from build123d import *

# Parameters (mm, degrees)
SKETCH_W        = 55
SKETCH_H        = 20
PAD_DEPTH       = 10
SKETCH001_W     = 50.5
SKETCH001_H     = 4.5
POCKET_DEPTH    = 18
SKETCH002_R     = 2.5
POCKET001_DEPTH = 5
SKETCH003_W     = 10
SKETCH003_H     = 10
PAD001_DEPTH    = 80
SKETCH004_W     = 10
SKETCH004_H     = 5
PAD002_DEPTH    = 13
SKETCH005_W     = 10
SKETCH005_H     = 5
PAD003_DEPTH    = 13
SKETCH006_W     = 5
SKETCH006_H     = 5
PAD004_DEPTH    = 23
SKETCH007_W     = 5
SKETCH007_H     = 5
PAD005_DEPTH    = 23
SKETCH008_W     = 5
SKETCH008_H     = 5
PAD006_DEPTH    = 15
SKETCH009_W     = 5
SKETCH009_H     = 5
PAD007_DEPTH    = 15


with BuildPart() as part:
    # Sketch → Pad (new body)
    with BuildSketch(Plane.XY):
        Rectangle(SKETCH_W, SKETCH_H)
    extrude(amount=PAD_DEPTH)

    # Sketch001 (on Face3 of Pad) → Pocket (cut)
    with BuildSketch(Plane.XZ.offset(10)):
        with Locations((0, 5.069511)):
            Rectangle(SKETCH001_W, SKETCH001_H)
    extrude(amount=-POCKET_DEPTH, mode=Mode.SUBTRACT)

    # Sketch002 (on Face5 of Pocket) → Pocket001 (cut)
    with BuildSketch(Plane.XY.offset(10)):
        with Locations((0, -5.825869)):
            Circle(SKETCH002_R)
    extrude(amount=-POCKET001_DEPTH, mode=Mode.SUBTRACT)

    # Sketch003 (on Face4 of Pocket001) → Pad001 (join)
    with BuildSketch(Plane(origin=(0, 0, 0), x_dir=(1, 0, 0), z_dir=(0, 0, -1))):
        with Locations((0, 4.349566)):
            Rectangle(SKETCH003_W, SKETCH003_H)
    extrude(amount=PAD001_DEPTH)

    # Sketch004 (on Face7 of Pad001) → Pad002 (join)
    with BuildSketch(Plane(origin=(-5, 0, 0), x_dir=(0, -1, 0), z_dir=(-1, 0, 0))):
        with Locations((4.349566, -77.5)):
            Rectangle(SKETCH004_W, SKETCH004_H)
    extrude(amount=PAD002_DEPTH)

    # Sketch005 (on Face9 of Pad002) → Pad003 (join)
    with BuildSketch(Plane.YZ.offset(5)):
        with Locations((-4.349566, -77.5)):
            Rectangle(SKETCH005_W, SKETCH005_H)
    extrude(amount=PAD003_DEPTH)

    # Sketch006 (on Face21 of Pad003) → Pad004 (join)
    with BuildSketch(Plane.XZ.offset(9.349566)):
        with Locations((-15.5, -77.5)):
            Rectangle(SKETCH006_W, SKETCH006_H)
    extrude(amount=PAD004_DEPTH)

    # Sketch007 (on Face22 of Pad004) → Pad005 (join)
    with BuildSketch(Plane.XZ.offset(9.349566)):
        with Locations((15.5, -77.5)):
            Rectangle(SKETCH007_W, SKETCH007_H)
    extrude(amount=PAD005_DEPTH)

    # Sketch008 (on Face24 of Pad005) → Pad006 (join)
    with BuildSketch(Plane.XY.offset(-75)):
        with Locations((-15.5, -29.849566)):
            Rectangle(SKETCH008_W, SKETCH008_H)
    extrude(amount=PAD006_DEPTH)

    # Sketch009 (on Face29 of Pad006) → Pad007 (join)
    with BuildSketch(Plane.XY.offset(-75)):
        with Locations((15.5, -29.849566)):
            Rectangle(SKETCH009_W, SKETCH009_H)
    extrude(amount=PAD007_DEPTH)


solid = part.part
Geometry: final body of the model. Coordinates: model frame, mm. A direction names the side the tool comes from. Give positions to 0.01 mm unless a question says otherwise; leave off trailing zeros. Write each loop counter-clockwise with the first axis right and the second up, starting at its lowest first coordinate (ties: lowest second). Pieces come first, ordered by that corner, then holes. Notation, with made-up numbers: (85, 42) -> (114, 42) arc R26 ccw to (114, 57) -> close; hole circle Ø5 at (71.5, -18.5). An arc over 180 degrees is marked (long way). Answer as a JSON object with one key per item and string values.
1. Cut plane A-A on x = -14. Output: boundary loops of the cut face in (y, z).
Ans:
{"outline": "(-32.35, -80) -> (0.65, -80) -> (0.65, -75) -> (-27.35, -75) -> (-27.35, -60) -> (-32.35, -60) -> close; (-10, 0) -> (10, 0) -> (10, 10) -> (-10, 10) -> (-10, 7.32) -> (8, 7.32) -> (8, 2.82) -> (-10, 2.82) -> close"}
2. Access query for faces 4 (the flat face through (-14, -10, -75)), 5 (the flat face through (-25.25, -1, 5)), 6 (the flat face through (-5, -4, -37)), 7 (the flat face through (-18, -19.6, -75.2)). Directions: +Z, -Z, +X, -X, +Y, -Y. A direction counts if a zero-diameter tool reaches every point of the face in a straight line with its end or side. Return the directions, or none.
Ans:
{"face 4": "-X, +Y", "face 5": "-Y", "face 6": "-X, +Y, -Y", "face 7": "-Z, -X, +Y, -Y"}
3. Cut plane B-B on z = -63. Output: boundary loops of the cut face in (x, y).
Ans:
{"outline": "(-18, -32.35) -> (-13, -32.35) -> (-13, -27.35) -> (-18, -27.35) -> close; (-5, -9.35) -> (5, -9.35) -> (5, 0.65) -> (-5, 0.65) -> close; (13, -32.35) -> (18, -32.35) -> (18, -27.35) -> (13, -27.35) -> close"}
4. Contact query for flat-ended pins moving along their axis: pin 1 (10 mm diameter, centred on y = -21, z = -72.5, fed in from +X); pin 2 (2 mm diameter, centred on x = -19, y = 4.5, fed in from -Z); pin 3 (13 mm diameter, centred on x = -4, z = -48.5, fed in from -Y). Output: stop coordinate, or through.
Ans:
{"pin 1": "stops at x = 18", "pin 2": "stops at z = 0", "pin 3": "stops at y = -9.35"}
5. Mould query, pull axis Z, two halves, no side actions, for faces 1 (the flat face through (0, 8, 5)), 2 (the flat face through (0, -9.35, -49)), 3 (the flat face through (0, 0, 10)). Classes: pulls with the +Z half, pulls with the -Z half, needs draft (parallel to the pull), parting line crosses it, or undercut.
Ans:
{"face 1": "undercut", "face 2": "needs draft", "face 3": "pulls with the +Z half"}
6. Ray query, probe 1 along Z at (x, y) = (8, -2.5); probe 2 along Z at (x, y) = (-1, -3); probe 3 along Y at (x, z) = (0, 8). Return the intervals inside material, ascending. Write a range as from..to.
Ans:
{"probe 1": "z = -80..-75, 0..2.82, 7.32..10", "probe 2": "z = -80..2.82, 7.32..10", "probe 3": "y = -10..-8.33, -3.33..10"}
7. Cut plane C-C on y = -24.5. Output: boundary loops of the cut face in (x, z).
Ans:
{"outline": "(-18, -80) -> (-13, -80) -> (-13, -75) -> (-18, -75) -> close; (13, -80) -> (18, -80) -> (18, -75) -> (13, -75) -> close"}
8. Cut plane D-D on x = 21. Output: boundary loops of the cut face in (y, z), and give its area (3 significant figures).
Ans:
{"outline": "(-10, 0) -> (10, 0) -> (10, 10) -> (-10, 10) -> (-10, 7.32) -> (8, 7.32) -> (8, 2.82) -> (-10, 2.82) -> close", "area": "119 mm^2"}
